Design review of the part built by this model. Coordinates are the model's own, in mm. A direction names the side the tool comes from. Give positions to 0.01 mm unless a question says otherwise; leave off trailing zeros. Write each loop counter-clockwise with the first axis right and the second up, starting at its lowest first coordinate (ties: lowest second). Pieces come first, ordered by that corner, then holes.
```python
from build123d import *

# Parameters (mm, degrees)
F0_R      = 88.9
F0_R_2    = 177.8
F1_DEPTH  = 635
F3_DEPTH  = 254
F4_R      = 165.1
F5_DEPTH  = 254.001
F6_W      = 914.4
F6_H      = 889
F7_DEPTH  = 762.001
F8_R      = 177.8
F9_DEPTH  = 635.001
F10_W     = 762
F10_H     = 76.2
F11_DEPTH = 2032.001
F12_W     = 1270
F12_H     = 254
F13_DEPTH = 254
F15_DEPTH = 254


with BuildPart() as f1:
    # F0 (on Front) → F1 (new body, symmetric)
    with BuildSketch(Plane.XZ):
        with BuildLine():
            Line((0, 127), (0, 0))
            Line((0, 0), (1397, 0))
            Line((1397, 0), (1397, 254))
            Line((1397, 254), (762, 254))
            Line((762, 254), (762, 1016))
            ThreePointArc((762, 1016), (210.61162, 1356.77676), (152.4, 711.2))
            Line((152.4, 711.2), (152.4, 127))
            Line((152.4, 127), (0, 127))
        make_face()
        with Locations((457.2, 254)):
            Circle(F0_R, mode=Mode.SUBTRACT)
        with Locations((381, 1016)):
            Circle(F0_R_2, mode=Mode.SUBTRACT)
    extrude(amount=F1_DEPTH, both=True)

    # F2 (on face) → F3 (join)
    with BuildSketch(Plane.XY.offset(254)):
        with BuildLine():
            ThreePointArc((1397, 635), (762, 0), (1397, -635))
            Line((1397, -635), (1397, 635))
        make_face()
        with BuildLine():
            Line((1397, 635), (1397, -635))
            ThreePointArc((1397, -635), (1846.012806, -449.012806), (2032, 0))
            ThreePointArc((2032, 0), (1846.012806, 449.012806), (1397, 635))
        make_face()
    extrude(amount=-F3_DEPTH)

    # F4 (on face) → F5 (cut, through all)
    with BuildSketch(Plane.XY.offset(254)):
        with Locations((1397, 0)):
            Circle(F4_R)
    extrude(amount=-F5_DEPTH, mode=Mode.SUBTRACT)

    # F6 (on face) → F7 (cut, through all)
    with BuildSketch(Plane.YZ.offset(762)):
        with Locations((0, 1079.5)):
            Rectangle(F6_W, F6_H)
    extrude(amount=-F7_DEPTH, mode=Mode.SUBTRACT)

    # F8 (on face) → F9 (cut, through all)
    with BuildSketch(Plane.XY.offset(635)):
        with Locations((431.8, 0)):
            Circle(F8_R)
    extrude(amount=-F9_DEPTH, mode=Mode.SUBTRACT)

    # F10 (on face) → F11 (cut, through all)
    with BuildSketch(Plane(origin=(0, 0, 0), x_dir=(0, -1, 0), z_dir=(-1, 0, 0))):
        with Locations((0, 38.1)):
            Rectangle(F10_W, F10_H)
    extrude(amount=-F11_DEPTH, mode=Mode.SUBTRACT)

    # F12 (on face) → F13 (join)
    with BuildSketch(Plane.YZ.offset(762)):
        with Locations((0, 381)):
            Rectangle(F12_W, F12_H)
    extrude(amount=F13_DEPTH)

    # F14 (on face) → F15 (cut)
    with BuildSketch(Plane.YZ.offset(1016)):
        with BuildLine():
            ThreePointArc((254, 508), (0, 762), (-254, 508))
            Line((-254, 508), (254, 508))
        make_face()
        with BuildLine():
            Line((254, 508), (-254, 508))
            ThreePointArc((-254, 508), (0, 254), (254, 508))
        make_face()
    extrude(amount=-F15_DEPTH, mode=Mode.SUBTRACT)


solid = f1.part
```
(1) Consider section C-C, the plane z = 188. Give the boundary of the cut face in (x, y), then the cut area to 3 significant figures.
Resolved:
outline: (152.4, -635) - (397.64, -635) - (397.64, -174.49) arc R177.8 cw to (397.64, 174.49) - (397.64, 635) - (152.4, 635) - close; (516.76, -635) - (1397, -635) arc R635 ccw to (1397, 635) - (516.76, 635) - (516.76, 156.19) arc R177.8 cw to (516.76, -156.19) - close; hole circle Ø330.2 at (1397, 0)
area: 1,920,000 mm2
(2) Mouldability with a two-part tool opening along X and no side actions: class faces 1 (the face through (77, -9, 127)), 2 (the face through (1554.476, 49.592, 166.345)), 3 (the face through (220.385, 544.855, 1361.491)), 4 (the face through (254.172, 7.818, 359.512)) as pulls with the +X half, pulls with the -X half, needs draft (parallel to the pull), parting line crosses it, or undercut.
Resolved:
face 1: needs draft
face 2: undercut
face 3: parting line crosses it
face 4: undercut
(3) Consider section D-D, the plane z = 801. Give the boundary of the cut face in (x, y), then the cut area to 3 significant figures.
Resolved:
outline: (66.46, -635) - (762, -635) - (762, -457.2) - (66.46, -457.2) - close; (66.46, 457.2) - (762, 457.2) - (762, 635) - (66.46, 635) - close
area: 247,000 mm2
(4) Consider section B-B, the plane y = -61.5. Give the boundary of the cut face in (x, z).
Resolved:
outline: (0, 76.2) - (264.97, 76.2) - (264.97, 635) - (152.4, 635) - (152.4, 127) - (0, 127) - close; (598.63, 76.2) - (1243.78, 76.2) - (1243.78, 254) - (1016, 254) - (1016, 261.56) - (762, 261.56) - (762, 635) - (598.63, 635) - close; (1550.22, 76.2) - (2029.01, 76.2) - (2029.01, 254) - (1550.22, 254) - close
(5) To check wall thickness, follow L1, parallel to Y at x = 534, z = 1332.5; L2, parallel to Z at x = 457, y = 394; L3, parallel to Y at x = 431.8, z = 357. State the ranges of each line that lie inside material, in increasing order.
Resolved:
L1: y = -635 to -457.2, 457.2 to 635
L2: z = 0 to 165.1, 342.9 to 635
L3: y = -635 to -177.8, 177.8 to 635
(6) Tool access review of faces 5 (the face through (890.78, -5.59, 254.06)), 6 (the face through (939, 381, 38)), 7 (the face through (887, 442, 508)): name each direction out of +Z, -Z, +X, -X, +Y, -Y from which nothing blocks a thin tool from reaching the whole face with its end or side.
Resolved:
face 5: +Z, +X
face 6: -Z, +X, -X
face 7: +Z, +X, +Y, -Y
(7) Consider section A-A, the plane x = 884.5. Give the boundary of the cut face in (y, z), then the cut area to 3 significant figures.
Resolved:
outline: (-635, 0) - (-381, 0) - (-381, 76.2) - (381, 76.2) - (381, 0) - (635, 0) - (635, 508) - (254, 508) arc R254 cw to (-254, 508) - (-635, 508) - close
area: 486,000 mm2
(8) Clearance check with flat-ended pins moving along their axes: P1, Ø5, axis at y = 491, z = 491.5, coming from the -X side; P2, Ø4, axis at x = 1071.5, y = -289.5, coming from the -Z side; P3, Ø5, axis at x = 1311.5, y = 377, coming from the +Z side. State where each tip first meets the part, or that it passes through.
Resolved:
P1: stops at x = 152.4
P2: stops at z = 76.2
P3: stops at z = 254
